from build123d import *

# Parameters (mm, degrees)
F2_W      = 1400
F2_H      = 1400
F2_R      = 605
F3_DEPTH  = 5
F5_DEPTH  = 25
F6_R      = 158
F7_DEPTH  = 90
F8_R      = 180
F9_DEPTH  = 15
F10_R     = 20
F10_R_2   = 55
F11_DEPTH = 100
F12_R     = 60
F12_R_2   = 5.5
F13_DEPTH = 15
F14_R     = 16
F15_DEPTH = 500
F16_R     = 105
F16_R_2   = 9
F17_DEPTH = 25
F18_R     = 50
F19_DEPTH = 500
F20_R     = 31.5
F23_R     = 37.5
F24_DEPTH = 690
F25_R     = 80
F25_R_2   = 7
F26_DEPTH = 25
F27_R     = 32.5
F28_DEPTH = 500


with BuildPart() as f1:
    # F0 (on Front) → F1 (revolve)
    with BuildSketch(Plane.XZ):
        Polygon((0, 1014), (0, 0), (605, 0), (605, 1006), (613, 1006), (613, 1014), (605, 1014), align=None)
    revolve(axis=Axis((0, 0, 507), (0, 0, 1)))

    # F2 (on face) → F3 (join)
    with BuildSketch(Plane(origin=(0, 0, 0), x_dir=(1, 0, 0), z_dir=(0, 0, -1))):
        Rectangle(F2_W, F2_H)
        Circle(F2_R, mode=Mode.SUBTRACT)
        Circle(F2_R)
    extrude(amount=F3_DEPTH)

    # F4 (on face) → F5 (cut)
    with BuildSketch(Plane.XY):
        with BuildLine():
            Line((-550, 532), (-700, 532))
            Line((-700, 532), (-700, 432))
            Line((-700, 432), (-550, 432))
            ThreePointArc((-550, 432), (-535.857864, 437.857864), (-530, 452))
            Line((-530, 452), (-530, 512))
            ThreePointArc((-530, 512), (-535.857864, 526.142136), (-550, 532))
        make_face()
    extrude(amount=-F5_DEPTH, mode=Mode.SUBTRACT)

    # F6 (on face) → F7 (join)
    with BuildSketch(Plane.XY.offset(1014)):
        with Locations((-400, 0)):
            Circle(F6_R)
    extrude(amount=F7_DEPTH)

    # F8 (on face) → F9 (join)
    with BuildSketch(Plane.XY.offset(1104)):
        with Locations((-400, 0)):
            Circle(F8_R)
    extrude(amount=F9_DEPTH)

    # F10 (on face) → F11 (join)
    with BuildSketch(Plane.XY.offset(1014)):
        with Locations((0, 400)):
            Circle(F10_R)
        with Locations((0, -303)):
            Circle(F10_R_2)
    extrude(amount=F11_DEPTH)

    # F12 (on face) → F13 (join)
    with BuildSketch(Plane.XY.offset(1114)):
        with Locations((0, 400)):
            Circle(F12_R)
        with Locations((0, 355)):
            Circle(F12_R_2, mode=Mode.SUBTRACT)
        with Locations((-45, 400)):
            Circle(F12_R_2, mode=Mode.SUBTRACT)
        with Locations((45, 400)):
            Circle(F12_R_2, mode=Mode.SUBTRACT)
        with Locations((0, 445)):
            Circle(F12_R_2, mode=Mode.SUBTRACT)
    extrude(amount=-F13_DEPTH)

    # F14 (on face) → F15 (cut)
    with BuildSketch(Plane.XY.offset(1114)):
        with Locations((0, 400)):
            Circle(F14_R)
    extrude(amount=-F15_DEPTH, mode=Mode.SUBTRACT)

    # F16 (on face) → F17 (join)
    with BuildSketch(Plane.XY.offset(1114)):
        with Locations((0, -303)):
            Circle(F16_R)
        with Locations((-60.104076, -363.104076)):
            Circle(F16_R_2, mode=Mode.SUBTRACT)
        with Locations((0, -388)):
            Circle(F16_R_2, mode=Mode.SUBTRACT)
        with Locations((60.104076, -363.104076)):
            Circle(F16_R_2, mode=Mode.SUBTRACT)
        with Locations((-85, -303)):
            Circle(F16_R_2, mode=Mode.SUBTRACT)
        with Locations((-60.104076, -242.895924)):
            Circle(F16_R_2, mode=Mode.SUBTRACT)
        with Locations((85, -303)):
            Circle(F16_R_2, mode=Mode.SUBTRACT)
        with Locations((0, -218)):
            Circle(F16_R_2, mode=Mode.SUBTRACT)
        with Locations((60.104076, -242.895924)):
            Circle(F16_R_2, mode=Mode.SUBTRACT)
    extrude(amount=-F17_DEPTH)

    # F18 (on face) → F19 (cut)
    with BuildSketch(Plane.XY.offset(1114)):
        with Locations((0, -303)):
            Circle(F18_R)
    extrude(amount=-F19_DEPTH, mode=Mode.SUBTRACT)

    # F22: sweep along a path in F21
    with BuildLine(Plane.XZ) as f22_path:
        Line((400, 1014), (400, 1114))
        ThreePointArc((400, 1114), (470, 1184), (540, 1114))
    # F20 (on face) → F22 (sweep)
    with BuildSketch(Plane.XY.offset(1014)):
        with Locations((400, 0)):
            Circle(F20_R)
    sweep(path=f22_path.line)

    # F23 (on Right) → F24 (join)
    with BuildSketch(Plane.YZ):
        with Locations((0, 245)):
            Circle(F23_R)
    extrude(amount=F24_DEPTH)

    # F25 (on face) → F26 (join)
    with BuildSketch(Plane.YZ.offset(690)):
        with Locations((0, 245)):
            Circle(F25_R)
        with Locations((0, 180)):
            Circle(F25_R_2, mode=Mode.SUBTRACT)
        with Locations((-65, 245)):
            Circle(F25_R_2, mode=Mode.SUBTRACT)
        with Locations((65, 245)):
            Circle(F25_R_2, mode=Mode.SUBTRACT)
        with Locations((0, 310)):
            Circle(F25_R_2, mode=Mode.SUBTRACT)
    extrude(amount=-F26_DEPTH)

    # F27 (on face) → F28 (cut)
    with BuildSketch(Plane.YZ.offset(690)):
        with Locations((0, 245)):
            Circle(F27_R)
    extrude(amount=-F28_DEPTH, mode=Mode.SUBTRACT)


solid = f1.part
Geometry check sheet. Reference: the model listing, model coordinates, mm. A direction names the side the tool comes from. Coordinates: 2 decimals unless noted, no trailing zeros. Order: outer loops, then holes, each group sorted by start corner. A loop starts at its lowest first (then second) coordinate and runs counter-clockwise, first axis right, second up. Notation, with made-up numbers: (-22, 35.5) -> (-14, 35.5) arc R15 cw to (-14, 56.5) -> close; hole circle Ø5 at (61.25, -31.5). An arc over 180 degrees is marked (long way). Use a Markdown table: item, result. Add a question column.
1. Set-up check for faces 5 (the face through (540, 0, 1114)), 6 (the face through (-233.726, -68.941, 1111.395)), 7 (the face through (-401, -159, 1104)): record each of +Z, -Z, +X, -X, +Y, -Y from which the full face is reachable in a straight line by a thin tool's end or side.
2. Cross-section at C-C (z = 367.5). Enter the section's corners in (x, y), and give its area (3 significant figures).
3. Cross-section at A-A (y = -501). Enter the section's corners in (x, z), and give its area (3 significant figures).
4. Mould release check, pull along Y, two halves, no side actions. Record for faces 1 (the face through (-22.762, -405.503, 1101.675)), 2 (the face through (690, -1, 211)), 3 (the face through (-1, -302, 614)), 4 (the face through (430.045, 9.462, 1064.7)): pulls with the +Y half, pulls with the -Y half, needs draft (parallel to the pull), parting line crosses it, or undercut.
5. Material ranges on L1, parallel to Z at x = -580.5, y = 195.5; L2, parallel to Z at x = 69, y = -290; L3, parallel to Z at x = -210.5, y = 484.5, recorded low to high.
6. Go/stop test with flat-tipped pins: pin 1 Ø22.5 at (y, z) = (0, 180) entering from -X; pin 2 Ø8 at (x, z) = (-440.5, 675.5) entering from -Y; pin 3 Ø12 at (y, z) = (540, 1010.5) entering from +X. Record where each tip stops, or that it passes through.
7. Cross-section at D-D (y = 220). Enter the section's corners in (x, z), and give its area (3 significant figures).
8. Cross-section at B-B (x = 468.5). Give the number of separate pieces and of enclosed holes in the cut face, and give its area (3 significant figures).
Filled sheet:
| question | item | result |
|---|---|---|
| 1 | face 5 | +X, +Y, -Y |
| 1 | face 6 | +Z |
| 1 | face 7 | none |
| 2 | outline | circle Ø1210 at (0, 0) |
| 2 | area | 1,150,000 mm2 |
| 3 | outline | (-700, -5) -> (700, -5) -> (700, 0) -> (339.15, 0) -> (339.15, 1006) -> (353.23, 1006) -> (353.23, 1014) -> (-353.23, 1014) -> (-353.23, 1006) -> (-339.15, 1006) -> (-339.15, 0) -> (-700, 0) -> close |
| 3 | area | 695,000 mm2 |
| 4 | face 1 | undercut |
| 4 | face 2 | needs draft |
| 4 | face 3 | undercut |
| 4 | face 4 | parting line crosses it |
| 5 | L1 | -5 to 0, 1006 to 1014 |
| 5 | L2 | -5 to 1014, 1089 to 1114 |
| 5 | L3 | -5 to 1014 |
| 6 | pin 1 | x = -605 |
| 6 | pin 2 | y = -418.92 |
| 6 | pin 3 | x = 301.02 |
| 7 | outline | (-700, -5) -> (700, -5) -> (700, 0) -> (563.58, 0) -> (563.58, 1006) -> (572.16, 1006) -> (572.16, 1014) -> (-572.16, 1014) -> (-572.16, 1006) -> (-563.58, 1006) -> (-563.58, 0) -> (-700, 0) -> close |
| 7 | area | 1,150,000 mm2 |
| 8 | separate pieces | 2 |
| 8 | enclosed holes | 1 |
| 8 | area | 783,000 mm2 |
